Could you check a few things on this model? Use its own coordinates, in mm. A direction names the side the tool comes from. Give positions to 0.01 mm unless a question says otherwise; leave off trailing zeros. Loops run counter-clockwise (first coordinate to the right, second up) from the corner with the lowest first, then second, coordinate; pieces in that order, holes last. Notation, with made-up numbers: (-20, 15.25) - (0, 15.25) arc R33 ccw to (0, 43.25) - close; hole circle Ø5 at (81.5, 58.5). An arc over 180 degrees is marked (long way). Write each question's results on one line, items separated by ' | '. Start each with the question number.
```python
from build123d import *

# Parameters (mm, degrees)
EXTRUDE_1_DEPTH          = 10
CUT_EXTRUDE_1_DEPTH      = 252.652538235
CUT_EXTRUDE_1_DEPTH_BACK = 252.652538235
SKETCH_7_R               = 3.5
CUT_EXTRUDE_5_DEPTH      = 252.652538235
SKETCH_8_R               = 5
CUT_EXTRUDE_6_DEPTH      = 3
SKETCH_9_R               = 3
CUT_EXTRUDE_7_DEPTH      = 252.652538235
CUT_EXTRUDE_START        = -10
SKETCH_11_R              = 27
CUT_EXTRUDE_9_DEPTH      = 10
SKETCH_12_R              = 30
CUT_EXTRUDE_10_DEPTH     = 10
SKETCH_14_R              = 1.45
CUT_EXTRUDE_12_DEPTH     = 300
CHAMFER_1_SIZE           = 16.633608268
CHAMFER_1_SIZE_2         = 2
CHAMFER_1_SIZE_3         = 1.419352868
CHAMFER_1_SIZE_4         = 1.457737974
CHAMFER_1_SIZE_5         = 2.415237377
CHAMFER_1_SIZE_6         = 1.523154621
CHAMFER_1_SIZE_7         = 3.004873211
SKETCH_15_R              = 5.25
SKETCH_15_R_2            = 3.5
CUT_EXTRUDE_13_DEPTH     = 3


with BuildPart() as part:
    # 草图1 → 凸台-拉伸1 (new body)
    with BuildSketch(Plane.XY):
        with BuildLine():
            Line((0, 12.5), (199.067804112, 12.5))
            ThreePointArc((199.067804112, 12.5), (250, 0), (199.067804112, -12.5))
            Line((199.067804112, -12.5), (0, -12.5))
            ThreePointArc((0, -12.5), (-12.5, 0), (0, 12.5))
        make_face()
    extrude(amount=EXTRUDE_1_DEPTH)

    # 草图3 → 切除-拉伸1 (cut, two sides: drawn at the far end of the back side and taken through both)
    with BuildSketch(Plane.XY.offset(10).offset(-CUT_EXTRUDE_1_DEPTH_BACK)):
        Polygon((176.376805713, 7.5), (151.73545401, 7.5), (164.376805713, -7.5), (176.376805713, -7.5), align=None)
        Polygon((159.145761472, -7.5), (146.504409769, 7.5), (146.399203355, 7.5), (121.399203355, -7.5), align=None)
        Polygon((113.624600829, -7.5), (138.624600829, 7.5), (100.983249125, 7.5), align=None)
        Polygon((70.646998471, -7.5), (108.393556588, -7.5), (95.752204884, 7.5), (95.646998471, 7.5), align=None)
        Polygon((50.231044241, 7.5), (62.872395944, -7.5), (87.872395944, 7.5), align=None)
        Polygon((10, -7.5), (57.641351703, -7.5), (45, 7.5), align=None)
        with BuildLine():
            Line((34.845635859, 7.5), (10, 7.5))
            ThreePointArc((10, 7.5), (12.156331085, 2.910947362), (12.312475569, -2.157068696))
            Line((12.312475569, -2.157068696), (34.845635859, 7.5))
        make_face()
    extrude(amount=CUT_EXTRUDE_1_DEPTH + CUT_EXTRUDE_1_DEPTH_BACK, mode=Mode.SUBTRACT)

    # 草图7 → 切除-拉伸5 (cut, through all)
    with BuildSketch(Plane(origin=(0, 0, 0), x_dir=(-1, 0, 0), z_dir=(0, 0, -1))):
        Circle(SKETCH_7_R)
    extrude(amount=-CUT_EXTRUDE_5_DEPTH, mode=Mode.SUBTRACT)

    # 草图8 → 切除-拉伸6 (cut)
    with BuildSketch(Plane(origin=(0, 0, 0), x_dir=(-1, 0, 0), z_dir=(0, 0, -1))):
        with Locations((-223, 0)):
            Circle(SKETCH_8_R)
    extrude(amount=-CUT_EXTRUDE_6_DEPTH, mode=Mode.SUBTRACT)

    # 草图9 → 切除-拉伸7 (cut, through all)
    with BuildSketch(Plane(origin=(0, 0, 0), x_dir=(-1, 0, 0), z_dir=(0, 0, -1))):
        with Locations((-223, 0)):
            Circle(SKETCH_9_R)
    extrude(amount=-CUT_EXTRUDE_7_DEPTH, mode=Mode.SUBTRACT)

    # 草图11 → 切除-拉伸9 (cut)
    with BuildSketch(Plane.XY.offset(10).offset(CUT_EXTRUDE_START)):
        with Locations((223, 0)):
            Circle(SKETCH_11_R)
    extrude(amount=CUT_EXTRUDE_9_DEPTH, mode=Mode.SUBTRACT)

    # 草图12 → 切除-拉伸10 (cut)
    with BuildSketch(Plane.XY.offset(10)):
        with Locations((226, 0)):
            Circle(SKETCH_12_R)
    extrude(amount=-CUT_EXTRUDE_10_DEPTH, mode=Mode.SUBTRACT)

    # 草图14 → 切除-拉伸12 (cut)
    with BuildSketch(Plane.XY.offset(10)):
        with Locations((184.5, 4)):
            Circle(SKETCH_14_R)
        with Locations((189.5, 4)):
            Circle(SKETCH_14_R)
        with Locations((189.5, -4)):
            Circle(SKETCH_14_R)
        with Locations((184.5, -4)):
            Circle(SKETCH_14_R)
    extrude(amount=-CUT_EXTRUDE_12_DEPTH, mode=Mode.SUBTRACT)

    # 倒角1
    # the kernel refuses this chamfer: 16.633608268, 3.004873211, 2.415237377, 2, 1.523154621, 1.457737974, 1.419352868 mm, written as the material it adds along each edge
    with BuildSketch(Plane(origin=(164.376805713, -7.5, 0), x_dir=(0.9999946519205123, -0.0032704939035876055, 0), z_dir=(0, 0, 1))) as chamfer_1_piece_1:
        Polygon((CHAMFER_1_SIZE * 0.999994651904, CHAMFER_1_SIZE * 0.00327049390353), (-CHAMFER_1_SIZE_2 * 0.646924574173, CHAMFER_1_SIZE_2 * 0.762553995026), (0, 0), align=None)
    extrude(amount=10)
    with BuildSketch(Plane(origin=(151.73545401, 7.5, 0), x_dir=(0.9996219169112968, 0.027495876610586605, 0), z_dir=(0, 0, 1))) as chamfer_1_piece_2:
        Polygon((CHAMFER_1_SIZE_2 * 0.999621916911, -CHAMFER_1_SIZE_2 * 0.0274958766106), (CHAMFER_1_SIZE_3 * 0.623158385834, -CHAMFER_1_SIZE_3 * 0.782095662754), (0, 0), align=None)
    extrude(amount=10)
    with BuildSketch(Plane(origin=(159.145761472, -7.5, 10), x_dir=(-0.9996219169112968, -0.02749587661058747, 0), z_dir=(0, 0, -1))) as chamfer_1_piece_3:
        Polygon((CHAMFER_1_SIZE_2 * 0.999621916911, CHAMFER_1_SIZE_2 * 0.0274958766106), (CHAMFER_1_SIZE_3 * 0.623158385834, CHAMFER_1_SIZE_3 * 0.782095662754), (0, 0), align=None)
    extrude(amount=10)
    with BuildSketch(Plane(origin=(121.399203355, -7.5, 10), x_dir=(0.9985473741645164, -0.05388080872768336, 0), z_dir=(0, 0, -1))) as chamfer_1_piece_4:
        Polygon((CHAMFER_1_SIZE_4 * 0.998547373967, -CHAMFER_1_SIZE_4 * 0.053880808717), (CHAMFER_1_SIZE_2 * 0.828525861946, -CHAMFER_1_SIZE_2 * 0.559950797917), (0, 0), align=None)
    extrude(amount=10)
    with BuildSketch(Plane(origin=(113.624600829, -7.5, 10), x_dir=(-0.6693179531686358, 0.7429760948820275, 0), z_dir=(0, 0, -1))) as chamfer_1_piece_5:
        Polygon((CHAMFER_1_SIZE_2 * 0.999455005814, CHAMFER_1_SIZE_2 * 0.033010473375), (-CHAMFER_1_SIZE_5 * 0.191677362679, CHAMFER_1_SIZE_5 * 0.981457991195), (0, 0), align=None)
    extrude(amount=10)
    with BuildSketch(Plane(origin=(138.624600829, 7.5, 0), x_dir=(-0.9985473741645164, 0.05388080872768389, 0), z_dir=(0, 0, 1))) as chamfer_1_piece_6:
        Polygon((CHAMFER_1_SIZE_4 * 0.998547373967, CHAMFER_1_SIZE_4 * 0.053880808717), (CHAMFER_1_SIZE_2 * 0.828525861946, CHAMFER_1_SIZE_2 * 0.559950797917), (0, 0), align=None)
    extrude(amount=10)
    with BuildSketch(Plane(origin=(100.983249125, 7.5, 10), x_dir=(0.6007510451121151, -0.7994361649291964, 0), z_dir=(0, 0, -1))) as chamfer_1_piece_7:
        Polygon((CHAMFER_1_SIZE_3 * 0.998441703797, -CHAMFER_1_SIZE_3 * 0.0558046920381), (CHAMFER_1_SIZE_2 * 0.600751045112, -CHAMFER_1_SIZE_2 * 0.799436164929), (0, 0), align=None)
    extrude(amount=10)
    with BuildSketch(Plane(origin=(70.646998471, -7.5, 0), x_dir=(0.8430222103307435, 0.537878752963033, 0), z_dir=(0, 0, 1))) as chamfer_1_piece_8:
        Polygon((CHAMFER_1_SIZE_2 * 0.999621916911, -CHAMFER_1_SIZE_2 * 0.0274958766106), (CHAMFER_1_SIZE_4 * 0.843022210164, -CHAMFER_1_SIZE_4 * 0.537878752857), (0, 0), align=None)
    extrude(amount=10)
    with BuildSketch(Plane(origin=(108.393556588, -7.5, 0), x_dir=(-0.6007510451121131, 0.799436164929198, 0), z_dir=(0, 0, 1)), Plane(origin=(50.231044241, 7.5, 0), x_dir=(0.6007510451121165, -0.7994361649291954, 0), z_dir=(0, 0, 1)), Plane(origin=(57.641351703, -7.5, 0), x_dir=(-0.6007510451121163, 0.7994361649291957, 0), z_dir=(0, 0, 1))) as chamfer_1_piece_9:
        Polygon((CHAMFER_1_SIZE_3 * 0.998441703797, CHAMFER_1_SIZE_3 * 0.0558046920381), (CHAMFER_1_SIZE_2 * 0.600751045112, CHAMFER_1_SIZE_2 * 0.799436164929), (0, 0), align=None)
    extrude(amount=10)
    with BuildSketch(Plane(origin=(87.872395944, 7.5, 10), x_dir=(-0.8430222103307434, -0.5378787529630333, 0), z_dir=(0, 0, -1))) as chamfer_1_piece_10:
        Polygon((CHAMFER_1_SIZE_2 * 0.999621916911, CHAMFER_1_SIZE_2 * 0.0274958766106), (CHAMFER_1_SIZE_4 * 0.843022210164, CHAMFER_1_SIZE_4 * 0.537878752857), (0, 0), align=None)
    extrude(amount=10)
    with BuildSketch(Plane(origin=(62.872395944, -7.5, 10), x_dir=(0.8689411613860879, 0.4949154049420938, 0), z_dir=(0, 0, -1))) as chamfer_1_piece_11:
        Polygon((CHAMFER_1_SIZE_5 * 0.99974277381, -CHAMFER_1_SIZE_5 * 0.0226800806836), (-CHAMFER_1_SIZE_2 * 0.18152448307, -CHAMFER_1_SIZE_2 * 0.983386425596), (0, 0), align=None)
    extrude(amount=10)
    with BuildSketch(Plane(origin=(10, -7.5, 10), x_dir=(0.9079663603978809, 0.419043062686671, 0), z_dir=(0, 0, -1))) as chamfer_1_piece_12:
        Polygon((CHAMFER_1_SIZE_2 * 0.999621916911, CHAMFER_1_SIZE_2 * 0.0274958766106), (CHAMFER_1_SIZE_6 * 0.907966360501, CHAMFER_1_SIZE_6 * 0.419043062734), (0, 0), align=None)
    extrude(amount=10)
    with BuildSketch(Plane(origin=(45, 7.5, 10), x_dir=(-0.9261548899255846, -0.3771433677886015, 0), z_dir=(0, 0, -1))) as chamfer_1_piece_13:
        Polygon((CHAMFER_1_SIZE_7 * 0.999834715095, -CHAMFER_1_SIZE_7 * 0.0181808325096), (-CHAMFER_1_SIZE_2 * 0.308450800004, -CHAMFER_1_SIZE_2 * 0.951240297705), (0, 0), align=None)
    extrude(amount=10)
    with BuildSketch(Plane(origin=(34.845635859, 7.5, 0), x_dir=(-0.9987654472434115, 0.0496747560906775, 0), z_dir=(0, 0, 1))) as chamfer_1_piece_14:
        Polygon((CHAMFER_1_SIZE_6 * 0.998765447357, CHAMFER_1_SIZE_6 * 0.0496747560963), (CHAMFER_1_SIZE_2 * 0.898442451911, CHAMFER_1_SIZE_2 * 0.439091289601), (0, 0), align=None)
    extrude(amount=10)

    # 草图15 → 切除-拉伸13 (cut)
    with BuildSketch(Plane(origin=(0, 0, 0), x_dir=(-1, 0, 0), z_dir=(0, 0, -1))):
        Circle(SKETCH_15_R)
        Circle(SKETCH_15_R_2, mode=Mode.SUBTRACT)
    extrude(amount=-CUT_EXTRUDE_13_DEPTH, mode=Mode.SUBTRACT)


solid = part.part
```
Q1. I'm going to push flat-ended pins straight in: pin 1 Ø6.5 at (x, y) = (0, 0) entering from +Z; pin 2 Ø3 at (x, y) = (-2.5, -2) entering from -Z; pin 3 Ø8 at (x, y) = (90, 0.5) entering from +Z; pin 4 Ø6 at (y, z) = (7, 6.5) entering from -X. Where does each tip first touch, or does it pass through?
Q2. Which directions (+Z, -Z, +X, -X, +Y, -Y) give clear straight access to the entire face, cutting with the end or side of a thin tool? Please do faces 1 (the face through (0, 4, 3)), 2 (the face through (101, -12.5, 5)), 3 (the face through (126.154, 0.018, 4.93)).
Q3. I want a section at B-B, the plane z = 7.25. State how many separate pieces and enclosed holes the cut face has, then the cut area to 3 significant figures.
Q4. I want a section at A-A, the plane x = 110.5. List the corners of the cut face in (y, z) for me, then the cut area to 3 significant figures.
Q5. If we mould it in two halves opening along Y, with no side actions, what happens to faces 4 (the face through (63.287, -6.116, 5.07)), 5 (the face through (98, 12.5, 5)), 6 (the face through (95, -8, 10))? For each: +Y half, -Y half, draft (parallel to the pull), parting line (faces both ways), or undercut.
Q6. I need wall thicknesses on L1, parallel to Y at x = 184.5, z = 4.5; L2, parallel to Y at x = 0, z = 5.75; L3, parallel to Y at x = 79, z = 3.5. Which ranges of each line are inside material? Lowest first, please. Write a range as from..to.
Conclusion:
1) pin 1: through | pin 2: z = 3 | pin 3: z = 10 | pin 4: x = -11.84
2) face 1: -Z | face 2: +Z, -Z, +X, -X, -Y | face 3: +Z, -Z
3) separate pieces: 1 | enclosed holes: 12 | area: 3,260 mm^2
4) outline: (-12.5, 0) - (-3.79, 0) - (-3.79, 10) - (-12.5, 10) - close; (7.5, 0) - (12.5, 0) - (12.5, 10) - (7.5, 10) - close | area: 137 mm^2
5) face 4: undercut | face 5: +Y half | face 6: draft
6) L1: -12.5..-5.45, -2.55..2.55, 5.45..12.5 | L2: -12.5..-3.5, 3.5..12.5 | L3: -12.5..-7.5, -2.49..2.18, 7.5..12.5
